Check sheet for the modelled part. Datum: model origin and axes. Units: mm. Coordinates: 2 decimals unless noted, no trailing zeros. Loops run counter-clockwise (first coordinate to the right, second up) from the corner with the lowest first, then second, coordinate; pieces in that order, holes last. Notation, with made-up numbers: M 86,48 L 92,48 A17 ccw 92,75 Z; hole C 25,65 d10. An arc over 180 degrees is marked long. Answer as CSV lines item,"result". Start each with the question number.
from build123d import *

# Parameters (mm, degrees)
F2_R = 1
F3_R = 1


with BuildPart() as f1:
    # F0 (on Front) → F1 (revolve)
    with BuildSketch(Plane.XZ):
        Polygon((-28, 50), (-28, 0), (-19, 0), (-19, 50), (-27.5, 80), (-35.5, 80), align=None)
    revolve(axis=Axis((0, 0, 61.423291), (0, 0, 1)))

    # F2
    f2_edges = [f1.edges().sort_by_distance(p)[0] for p in [
        (27.5, 0, 80),
    ]]
    fillet(f2_edges, radius=F2_R)

    # F3
    f3_edges = [f1.edges().sort_by_distance(p)[0] for p in [
        (35.5, 0, 80),
        (28, 0, 0),
        (19, 0, 0),
    ]]
    fillet(f3_edges, radius=F3_R)


solid = f1.part
Item 1: Release check for a two-part mould opening along X. For faces 1 (the face through (5, -28, 80)), 2 (the face through (-25.865, 10.724, 25.157)), 3 (the face through (-8.767, 16.856, 25.843)) record: released by +X, released by -X, zero draft, split by the parting line, or undercut.
Item 2: Sectioned sample at D-D, the plane z = 73.5. Record the boundary of the cut face in (x, y) (3 decimals).
Item 3: Sectioned sample at C-C, the plane z = 35. Record the boundary of the cut face in (x, y).
Item 4: Go/stop test with flat-tipped pins: pin 1 (8 mm diameter, centred on x = 17.5, z = 56.5, fed in from +Y); pin 2 (1 mm diameter, centred on y = 3.5, z = 44, fed in from -X); pin 3 (4 mm diameter, centred on y = -25, z = 27, fed in from +X). Record where each tip stops, or that it passes through.
Item 5: Material ranges on line 1 (Y direction, x = 0, z = 35.5); line 2 (X direction, y = -17, z = 52), recorded low to high. Write a range as from..to.
Item 6: Sectioned sample at A-A, the plane y = 0. Record the boundary of the cut face in (x, z), and give its area (3 significant figures).
Reply:
1,face 1,"zero draft"
1,face 2,"split by the parting line"
1,face 3,"undercut"
2,outline,"C 0,0 d67.75; hole C 0,0 d51.317"
3,outline,"C 0,0 d56; hole C 0,0 d38"
4,pin 1,"y = 26.66"
4,pin 2,"x = -27.84"
4,pin 3,"x = 15.97"
5,line 1,"-28..-19, 19..28"
5,line 2,"-22.87..-9.69, 9.69..22.87"
6,outline,"M -35.19,78.76 L -28,50 L -28,1 A1 ccw -27,0 L -20,0 A1 ccw -19,1 L -19,50 L -27.29,79.27 A1 ccw -28.26,80 L -34.22,80 A1 ccw Z; M 19,1 A1 ccw 20,0 L 27,0 A1 ccw 28,1 L 28,50 L 35.19,78.76 A1 ccw 34.22,80 L 28.26,80 A1 ccw 27.29,79.27 L 19,50 Z"
6,area,"1,410 mm²"
